Check sheet for the modelled part. Datum: model origin and axes. Units: mm. A direction names the side the tool comes from. Give positions to 0.01 mm unless a question says otherwise; leave off trailing zeros. Loops run counter-clockwise (first coordinate to the right, second up) from the corner with the lowest first, then second, coordinate; pieces in that order, holes last. Notation, with made-up numbers: (11, 60) - (57, 60) arc R30 cw to (57, 82) - close; hole circle Ø9 at (34, -14.5). An arc over 180 degrees is marked (long way). Answer in a Markdown table with one row per item. Add a question column.
(1) Set-up check for faces 1 (the face through (39.9, 11.4, 3.5)), 2 (the face through (20.07, 34.76, 3.06)): record each of +Z, -Z, +X, -X, +Y, -Y from which the full face is reachable in a straight line by a thin tool's end or side.
(2) Draft check along X on faces 3 (the face through (60.07, 34.52, 3.06)), 4 (the face through (18.236, 10.793, 3.944)), 5 (the face through (37, 38, 4)), 6 (the face through (55, 12, 8)). Enter one of: released by +X, released by -X, zero draft, split by the parting line, or undercut.
(3) Sectioned sample at D-D on y = 42. Enter the section's corners in (x, z).
(4) Go/stop test with flat-tipped pins: P1, Ø1.5, axis at x = 26.5, z = 2, coming from the -Y side; P2, Ø3.5, axis at x = 52.99, y = 15.59, coming from the +Z side; P3, Ø2, axis at x = 26, z = 2.5, coming from the -Y side. Record where each tip stops, or that it passes through.
(5) Sectioned sample at A-A on z = 6. Enter the section's corners in (x, y), then the cut area to 3 significant figures.
(6) Sectioned sample at B-B on z = 1. Enter the section's corners in (x, y), then the cut area to 3 significant figures.
(7) Sectioned sample at C-C on y = 10.5. Enter the section's corners in (x, z), then the cut area to 3 significant figures.
(8) Thickness scan on L1, parallel to Y at x = 52, z = 5; L2, parallel to X at y = 17.5, z = 1.25; L3, parallel to X at y = 31.5, z = 4.5. Record the ranges inside material, lowest first.
from build123d import *

# Parameters (mm, degrees)
F0_R     = 3
F1_DEPTH = 8
F2_R     = 4.5
F3_DEPTH = 23.2
F4_R     = 4.5
F5_DEPTH = 23.2
F6_R     = 4.5
F7_DEPTH = 23.2


with BuildPart() as f1:
    # F0 (on Top) → F1 (new body)
    with BuildSketch(Plane.XY):
        with BuildLine():
            Line((24.7871355388, 42.9325781273), (15.2128644612, 26.3494541755))
            ThreePointArc((15.2128644612, 26.3494541755), (18.3493649054, 10.5940107676), (30.4257289224, 0))
            Line((30.4257289224, 0), (49.5742710776, 0))
            ThreePointArc((49.5742710776, 0), (61.6506350946, 10.5940107676), (64.7871355388, 26.3494541755))
            Line((64.7871355388, 26.3494541755), (55.2128644612, 42.9325781273))
            ThreePointArc((55.2128644612, 42.9325781273), (40, 48.0940107676), (24.7871355388, 42.9325781273))
        make_face()
        with Locations((27.0096189432, 15.5940107676)):
            Circle(F0_R, mode=Mode.SUBTRACT)
        with Locations((52.9903810568, 15.5940107676)):
            Circle(F0_R, mode=Mode.SUBTRACT)
        with Locations((40, 38.0940107676)):
            Circle(F0_R, mode=Mode.SUBTRACT)
    extrude(amount=F1_DEPTH)

    # F2 (on face) → F3 (cut)
    with BuildSketch(Plane.XZ):
        with Locations((40, 8)):
            Circle(F2_R)
    extrude(amount=-F3_DEPTH, mode=Mode.SUBTRACT)

    # F4 (on face) → F5 (cut)
    with BuildSketch(Plane(origin=(60, 34.6410161514, 0), x_dir=(-0.5, 0.8660254038, 0), z_dir=(0.8660254038, 0.5, 0))):
        with Locations((0, 8)):
            Circle(F4_R)
    extrude(amount=-F5_DEPTH, mode=Mode.SUBTRACT)

    # F6 (on face) → F7 (cut)
    with BuildSketch(Plane(origin=(0, 0, 0), x_dir=(-0.5, -0.8660254038, 0), z_dir=(-0.8660254038, 0.5, 0))):
        with Locations((-40, 8)):
            Circle(F6_R)
    extrude(amount=-F7_DEPTH, mode=Mode.SUBTRACT)


solid = f1.part
Reply:
| question | item | result |
|---|---|---|
| 1 | face 1 | +Z, -Y |
| 1 | face 2 | +Z, -Z, -X, +Y |
| 2 | face 3 | released by +X |
| 2 | face 4 | released by -X |
| 2 | face 5 | undercut |
| 2 | face 6 | zero draft |
| 3 | outline | (24.25, 0) - (55.75, 0) - (55.75, 8) - (24.25, 8) - close |
| 4 | P1 | y = 1.59 |
| 4 | P2 | through |
| 4 | P3 | y = 1.74 |
| 5 | outline | (15.21, 26.35) arc R25 ccw to (30.43, 0) - (35.97, 0) - (35.97, 20.77) - (17.98, 31.15) - close; (22.02, 38.13) - (40, 27.75) - (57.98, 38.13) - (55.21, 42.93) arc R25 ccw to (24.79, 42.93) - close; (44.03, 0) - (49.57, 0) arc R25 ccw to (64.79, 26.35) - (62.02, 31.15) - (44.03, 20.77) - close; hole circle Ø6 at (27.01, 15.59); hole circle Ø6 at (40, 38.09); hole circle Ø6 at (52.99, 15.59) |
| 5 | area | 1,270 mm^2 |
| 6 | outline | (15.21, 26.35) arc R25 ccw to (30.43, 0) - (49.57, 0) arc R25 ccw to (64.79, 26.35) - (55.21, 42.93) arc R25 ccw to (24.79, 42.93) - close; hole circle Ø6 at (27.01, 15.59); hole circle Ø6 at (40, 38.09); hole circle Ø6 at (52.99, 15.59) |
| 6 | area | 1,810 mm^2 |
| 7 | outline | (18.4, 0) - (61.6, 0) - (61.6, 8) - (44.5, 8) arc R4.5 cw to (35.5, 8) - (18.4, 8) - close |
| 7 | area | 314 mm^2 |
| 8 | L1 | 1.16 to 12.76, 18.43 to 26.15, 33.9 to 45.03 |
| 8 | L2 | 15.63 to 24.69, 29.33 to 50.67, 55.31 to 64.37 |
| 8 | L3 | 18.19 to 19.78, 31.1 to 48.9, 60.22 to 61.81 |
